Part model, mm, in its own coordinate system. A direction names the side the tool comes from. Coordinates: 2 decimals unless noted, no trailing zeros. Loops run counter-clockwise (first coordinate to the right, second up) from the corner with the lowest first, then second, coordinate; pieces in that order, holes last. Notation, with made-up numbers: (10.5, 47) -> (51.5, 47) arc R15 cw to (51.5, 64) -> close; hole circle Ø3 at (0, 17.5). An arc over 180 degrees is marked (long way). One line per question, with ' | ' between items. Start each with the question number.
1) 3-axis set-ups, long thin cutter, end or side, ignore diameter. For faces 3 (the face through (-2, 13, 3)), 4 (the face through (0, 17, -4)): which of +Z, -Z, +X, -X, +Y, -Y reach the whole face in a straight line?
2) Probe L1, parallel to Y at x = 0, z = 3.75; L2, parallel to Y at x = 19.5, z = 5.5; L3, parallel to X at y = -12, z = 3. List the from-to ranges inside material, lowest first. Write a range as from..to.
3) Cut at A-A (y = 19). Count the separate pieces of the cut face and the enclosed holes in it, plus the area to 3 significant figures.
4) Cut at C-C (z = -7). List the corners of the cut face in (x, y), plus the area to 3 significant figures.
5) Two-plate mould, pull along Y, no slides. Class faces 1 (the face through (-12.56, -4.94, 2.55)), 2 (the face through (21, 14, 10)): released by +Y, released by -Y, zero draft, split by the parting line, or undercut.
6) Drop flat-ended pins along their axis: pin 1 (1 mm diameter, centred on y = -16, z = -1.5, fed in from -X); pin 2 (6 mm diameter, centred on y = -23, z = -3.5, fed in from -X); pin 3 (4 mm diameter, centred on y = -28.5, z = -2, fed in from +X); pin 4 (4 mm diameter, centred on x = 0, y = 20, fed in from +Z). Give the stop position or say it passes through.
from build123d import *

# Parameters (mm, degrees)
SKETCH_2_R               = 5.5
EXTRUDE_1_DEPTH          = 10
PATTERN_CIRCULAR_1_COUNT = 6
EXTRUDE_2_DEPTH          = 7
SKETCH_4_R               = 1.4
CUT_EXTRUDE_1_DEPTH      = 12
PATTERN_CIRCULAR_2_COUNT = 6
SKETCH_5_R               = 9
EXTRUDE_3_DEPTH          = 5
SKETCH_7_R               = 7
CUT_EXTRUDE_3_DEPTH      = 1.5
CUT_EXTRUDE_3_TAPER      = 40
SKETCH_8_R               = 1.5
CUT_EXTRUDE_4_DEPTH      = 15.5
SKETCH_10_R              = 1.25
CUT_EXTRUDE_6_DEPTH      = 17
SKETCH_11_R              = 2.5
CUT_EXTRUDE_7_DEPTH      = 17
PATTERN_CIRCULAR_4_COUNT = 6
CUT_EXTRUDE_9_DEPTH      = 8


with BuildPart() as part:
    # 草图1 → 旋转1 (revolve)
    with BuildSketch(Plane(origin=(0, 0, 0), x_dir=(1, 0, 0), z_dir=(0, 1, 0))):
        with BuildLine():
            Line((25, 10), (25, -10))
            Line((25, -10), (31, -10))
            ThreePointArc((31, -10), (35.787135539, -6.443375673), (33.763853992, -0.833333333))
            ThreePointArc((33.763853992, -0.833333333), (33.31662479, 0), (33.763853992, 0.833333333))
            ThreePointArc((33.763853992, 0.833333333), (35.787135539, 6.443375673), (31, 10))
            Line((31, 10), (25, 10))
        make_face()
    revolve(axis=Axis((0, 0, -146.934042126), (0, 0, 1)))

    # 草图2 → 凸台-拉伸1 (add)
    with BuildSketch(Plane.XY.offset(6)):
        with Locations((0, 20)):
            Circle(SKETCH_2_R)
    extrude_1 = extrude(amount=-EXTRUDE_1_DEPTH)

    # 阵列(圆周)1: 凸台-拉伸1 ×6 about axis
    pattern_circular_1_axis = Axis((0, 0, 0), (0, 0, 1))
    for i in range(1, PATTERN_CIRCULAR_1_COUNT):
        add(extrude_1.rotate(pattern_circular_1_axis, i * 360 / PATTERN_CIRCULAR_1_COUNT))

    # 草图3 → 凸台-拉伸2 (add)
    with BuildSketch(Plane.XY.offset(6)):
        with BuildLine():
            Line((-8.849844437, 0), (-11.274766656, -4.200088487))
            Line((-11.274766656, -4.200088487), (-13.883448238, -5.706211501))
            ThreePointArc((-13.883448238, -5.706211501), (-12.557368355, -7.25), (-11.883448238, -9.170313116))
            Line((-11.883448238, -9.170313116), (-9.274766656, -7.664190102))
            Line((-9.274766656, -7.664190102), (-4.424922219, -7.664190102))
            Line((-4.424922219, -7.664190102), (-2, -11.864278589))
            Line((-2, -11.864278589), (-2, -14.876524617))
            ThreePointArc((-2, -14.876524617), (0, -14.5), (2, -14.876524617))
            Line((2, -14.876524617), (2, -11.864278589))
            Line((2, -11.864278589), (4.424922219, -7.664190102))
            Line((4.424922219, -7.664190102), (9.274766656, -7.664190102))
            Line((9.274766656, -7.664190102), (11.883448238, -9.170313116))
            ThreePointArc((11.883448238, -9.170313116), (12.557368355, -7.25), (13.883448238, -5.706211501))
            Line((13.883448238, -5.706211501), (11.274766656, -4.200088487))
            Line((11.274766656, -4.200088487), (8.849844437, 0))
            Line((8.849844437, 0), (11.274766656, 4.200088487))
            Line((11.274766656, 4.200088487), (13.883448238, 5.706211501))
            ThreePointArc((13.883448238, 5.706211501), (12.557368355, 7.25), (11.883448238, 9.170313116))
            Line((11.883448238, 9.170313116), (9.274766656, 7.664190102))
            Line((9.274766656, 7.664190102), (4.424922219, 7.664190102))
            Line((4.424922219, 7.664190102), (2, 11.864278589))
            Line((2, 11.864278589), (2, 14.876524617))
            ThreePointArc((2, 14.876524617), (0, 14.5), (-2, 14.876524617))
            Line((-2, 14.876524617), (-2, 11.864278589))
            Line((-2, 11.864278589), (-4.424922219, 7.664190102))
            Line((-4.424922219, 7.664190102), (-9.274766656, 7.664190102))
            Line((-9.274766656, 7.664190102), (-11.883448238, 9.170313116))
            ThreePointArc((-11.883448238, 9.170313116), (-12.557368355, 7.25), (-13.883448238, 5.706211501))
            Line((-13.883448238, 5.706211501), (-11.274766656, 4.200088487))
            Line((-11.274766656, 4.200088487), (-8.849844437, 0))
        make_face()
    extrude(amount=-EXTRUDE_2_DEPTH)

    # 草图4 → 切除-拉伸1 (cut, through all)
    with BuildSketch(Plane(origin=(0, 0, -1), x_dir=(-1, 0, 0), z_dir=(0, 0, -1))):
        with Locations((0, 12)):
            Circle(SKETCH_4_R)
    cut_extrude_1 = extrude(amount=-CUT_EXTRUDE_1_DEPTH, mode=Mode.SUBTRACT)

    # 阵列(圆周)2: 切除-拉伸1 ×6 about axis
    pattern_circular_2_axis = Axis((0, 0, 0), (0, 0, 1))
    for i in range(1, PATTERN_CIRCULAR_2_COUNT):
        add(cut_extrude_1.rotate(pattern_circular_2_axis, i * 360 / PATTERN_CIRCULAR_2_COUNT), mode=Mode.SUBTRACT)

    # 草图5 → 凸台-拉伸3 (add)
    with BuildSketch(Plane(origin=(0, 0, -1), x_dir=(-1, 0, 0), z_dir=(0, 0, -1))):
        Circle(SKETCH_5_R)
    extrude(amount=EXTRUDE_3_DEPTH)

    # 草图7 → 切除-拉伸3 (cut)
    with BuildSketch(Plane.XY.offset(6)):
        Circle(SKETCH_7_R)
    extrude(amount=-CUT_EXTRUDE_3_DEPTH, taper=CUT_EXTRUDE_3_TAPER, mode=Mode.SUBTRACT)

    # 草图8 → 切除-拉伸4 (cut, through all)
    with BuildSketch(Plane.XY.offset(4.5)):
        Circle(SKETCH_8_R)
    extrude(amount=-CUT_EXTRUDE_4_DEPTH, mode=Mode.SUBTRACT)

    # 草图10 → 切除-拉伸6 (cut, through all)
    with BuildSketch(Plane.XY.offset(6)):
        with Locations((0, 20)):
            Circle(SKETCH_10_R)
    extrude(amount=-CUT_EXTRUDE_6_DEPTH, mode=Mode.SUBTRACT)

    # 草图11 → 切除-拉伸7 (cut, through all)
    with BuildSketch(Plane.XY.offset(6)):
        with Locations((0, 20)):
            Circle(SKETCH_11_R)
    cut_extrude_7 = extrude(amount=-CUT_EXTRUDE_7_DEPTH, mode=Mode.SUBTRACT)

    # 阵列(圆周)4: 切除-拉伸7 ×6 about axis
    pattern_circular_4_axis = Axis((0, 0, 0), (0, 0, 1))
    for i in range(1, PATTERN_CIRCULAR_4_COUNT):
        add(cut_extrude_7.rotate(pattern_circular_4_axis, i * 360 / PATTERN_CIRCULAR_4_COUNT), mode=Mode.SUBTRACT)

    # 草图14 → 切除-拉伸9 (cut)
    with BuildSketch(Plane(origin=(0, 0, -6), x_dir=(-1, 0, 0), z_dir=(0, 0, -1))):
        Polygon((0, 6.92820323), (-6, 3.464101615), (-6, -3.464101615), (0, -6.92820323), (6, -3.464101615), (6, 3.464101615), align=None)
    extrude(amount=-CUT_EXTRUDE_9_DEPTH, mode=Mode.SUBTRACT)


solid = part.part
Reported:
1) face 3: +Z, -Z | face 4: -Z
2) L1: y = -35.84..-22.5, -17.5..-13.4, -10.6..-1.5, 1.5..10.6, 13.4..17.5, 22.5..35.84 | L2: y = -30.23..-15.64, -15.05..-11.22, -8.78..-4.95, 4.95..8.78, 11.22..15.05, 15.64..30.23 | L3: x = -33.5..-18.82, -15.82..-12.2, -2..-1.4, 1.4..2, 12.2..15.82, 18.82..33.5
3) separate pieces: 4 | enclosed holes: 0 | area: 587 mm²
4) outline: circle Ø71.17 at (0, 0); hole circle Ø50 at (0, 0) | area: 2,010 mm²
5) face 1: undercut | face 2: zero draft
6) pin 1: stops at x = -31.2 | pin 2: stops at x = -29.8 | pin 3: stops at x = 23.44 | pin 4: passes through
